Work out the finished part from the listing and answer in its coordinate system (mm). A direction names the side the tool comes from. Coordinates: 2 decimals unless noted, no trailing zeros. Order: outer loops, then holes, each group sorted by start corner. A loop starts at its lowest first (then second) coordinate and runs counter-clockwise, first axis right, second up. Notation, with made-up numbers: (32, 78) -> (72, 78) arc R24 cw to (72, 93) -> close; hole circle Ø4 at (89.25, 60). An arc over 180 degrees is marked (long way). Use one line per item in the form item = value.
from build123d import *

# Parameters (mm, degrees)
SKETCH1_W           = 37
SKETCH1_H           = 22.5
BOSS_EXTRUDE1_DEPTH = 20
BOSS_EXTRUDE2_DEPTH = 25
SKETCH3_R           = 2.5
BOSS_EXTRUDE3_DEPTH = 9.1
SKETCH4_R           = 2.5
BOSS_EXTRUDE4_DEPTH = 9.1
FILLET1_R           = 3
FILLET2_R           = 4
SKETCH5_W           = 2.75
SKETCH5_H           = 5
BOSS_EXTRUDE5_DEPTH = 5
SKETCH6_R           = 1.5
CUT_EXTRUDE1_DEPTH  = 2.75
SKETCH7_R           = 1.5
CUT_EXTRUDE2_DEPTH  = 30.1
SKETCH8_W           = 8.509980697
SKETCH8_H           = 2.764975678
SKETCH8_W_2         = 9.677414873
SKETCH8_H_2         = 2.427034206
CUT_EXTRUDE3_DEPTH  = 8.9
SKETCH9_W           = 9.677414873
SKETCH9_H           = 2.427034206
SKETCH9_W_2         = 8.509980697
SKETCH9_H_2         = 2.764975678
CUT_EXTRUDE4_DEPTH  = 8.9


with BuildPart() as part:
    # Sketch1 → Boss-Extrude1 (new body)
    with BuildSketch(Plane.XY):
        with Locations((-45.764100782, -13.75)):
            Rectangle(SKETCH1_W, SKETCH1_H)
    extrude(amount=-BOSS_EXTRUDE1_DEPTH)

    # Sketch2 → Boss-Extrude2 (add)
    with BuildSketch(Plane(origin=(-27.264100782, 0, 0), x_dir=(0, 0, -1), z_dir=(1, 0, 0))):
        with BuildLine():
            ThreePointArc((0.050125629, -14), (10, -24.462429423), (19.949874371, -14))
            ThreePointArc((19.949874371, -14), (10, -3), (0.050125629, -14))
        make_face()
    extrude(amount=BOSS_EXTRUDE2_DEPTH)

    # Sketch3 → Boss-Extrude3 (add)
    with BuildSketch(Plane.XY):
        with Locations((-54.264100782, -14)):
            Circle(SKETCH3_R)
    extrude(amount=BOSS_EXTRUDE3_DEPTH)

    # Sketch4 → Boss-Extrude4 (add)
    with BuildSketch(Plane(origin=(0, 0, -20), x_dir=(-1, 0, 0), z_dir=(0, 0, -1))):
        with Locations((54.264100782, -14)):
            Circle(SKETCH4_R)
    extrude(amount=BOSS_EXTRUDE4_DEPTH)

    # Fillet1
    fillet1_edges = [part.edges().sort_by_distance(p)[0] for p in [
        (-64.264100782, -2.5, -10),
        (-64.264100782, -25, -10),
    ]]
    fillet(fillet1_edges, radius=FILLET1_R)

    # Fillet2
    fillet2_edges = [part.edges().sort_by_distance(p)[0] for p in [
        (-2.264100782, -3, -10),
        (-2.264100782, -24.462429423, -10),
    ]]
    fillet(fillet2_edges, radius=FILLET2_R)

    # Sketch5 → Boss-Extrude5 (add)
    with BuildSketch(Plane.ZY.offset(64.264100782)):
        with Locations((-10, -13.75)):
            Rectangle(SKETCH5_W, SKETCH5_H)
    extrude(amount=BOSS_EXTRUDE5_DEPTH)

    # Sketch6 → Cut-Extrude1 (cut)
    with BuildSketch(Plane(origin=(0, 0, -11.375), x_dir=(-1, 0, 0), z_dir=(0, 0, -1))):
        with Locations((66.764100782, -13.75)):
            Circle(SKETCH6_R)
    extrude(amount=-CUT_EXTRUDE1_DEPTH, mode=Mode.SUBTRACT)

    # Sketch7 → Cut-Extrude2 (cut, through all)
    with BuildSketch(Plane(origin=(0, 0, -20), x_dir=(-1, 0, 0), z_dir=(0, 0, -1))):
        with Locations((31.264100782, -5)):
            Circle(SKETCH7_R)
        with Locations((31.264100782, -23)):
            Circle(SKETCH7_R)
    extrude(amount=-CUT_EXTRUDE2_DEPTH, mode=Mode.SUBTRACT)

    # Sketch8 → Cut-Extrude3 (cut)
    with BuildSketch(Plane(origin=(0, 0, -29.1), x_dir=(-1, 0, 0), z_dir=(0, 0, -1))):
        with Locations((54.477604306, -17.132487839)):
            Rectangle(SKETCH8_W, SKETCH8_H)
        with Locations((54.323994545, -11.036482897)):
            Rectangle(SKETCH8_W_2, SKETCH8_H_2)
    extrude(amount=-CUT_EXTRUDE3_DEPTH, mode=Mode.SUBTRACT)

    # Sketch9 → Cut-Extrude4 (cut)
    with BuildSketch(Plane.XY.offset(9.1)):
        with Locations((-54.323994545, -11.036482897)):
            Rectangle(SKETCH9_W, SKETCH9_H)
        with Locations((-54.477604306, -17.132487839)):
            Rectangle(SKETCH9_W_2, SKETCH9_H_2)
    extrude(amount=-CUT_EXTRUDE4_DEPTH, mode=Mode.SUBTRACT)


solid = part.part
(1) Which of the six approach directions +Z, -Z, +X, -X, +Y, -Y give full straight-line access (tool end or side, diameter ignored) to faces 1 (the cylindrical face through (-51.767, -13.89, -24.486)), 2 (the flat face through (-54, -12.25, 5)), 3 (the flat face through (-54, -15.75, -25)), 4 (the flat face through (-54, -15.75, 5))?
Data:
face_1 = -Z
face_2 = +Z, +X, -X, +Y
face_3 = -Z, +X, -X, -Y
face_4 = +Z, +X, -X, -Y
(2) Straight lines are drawn through the part: line 1 along Z through (x, y) = (-34, -19.75); line 2 along X through (y, z) = (-14, -15); line 3 along X through (y, z) = (-22.25, -10.5). For each, find the intervals that lie inside material, in ascending order.
Data:
line_1 = -20 to 0
line_2 = -64.26 to -2.26
line_3 = -64.25 to -32.56, -29.97 to -2.69
(3) Section A-A on z = -10 is taken. Write down the section's boundary in (x, y), plus the area to 3 significant figures.
Data:
outline = (-69.26, -16.25) -> (-64.26, -16.25) -> (-64.26, -22) arc R3 ccw to (-61.26, -25) -> (-27.26, -25) -> (-27.26, -24.46) -> (-6.26, -24.46) arc R4 ccw to (-2.26, -20.46) -> (-2.26, -7) arc R4 ccw to (-6.26, -3) -> (-27.26, -3) -> (-27.26, -2.5) -> (-61.26, -2.5) arc R3 ccw to (-64.26, -5.5) -> (-64.26, -11.25) -> (-69.26, -11.25) -> close; hole circle Ø3 at (-66.76, -13.75); hole circle Ø3 at (-31.26, -23); hole circle Ø3 at (-31.26, -5)
area = 1,360 mm²
(4) Section D-D on x = -58 is taken. Write down the section's boundary in (y, z).
Data:
outline = (-25, -20) -> (-2.5, -20) -> (-2.5, 0) -> (-25, 0) -> close
(5) Each of these flat-tipped pins is pushed along its axis until it touches: P1, Ø0.6, axis at x = -54.5, y = -16, coming from the -Z side; P2, Ø10, axis at x = -14, y = -7.5, coming from the +Z side; P3, Ø10, axis at y = -11, z = 3, coming from the +X side; P4, Ø7, axis at x = -41, y = -13, coming from the -Z side. Where does it stop, or does it pass through?
Data:
P1 = -29.1
P2 = -0.01
P3 = -2.89
P4 = -20
(6) Section C-C on z = -19 is taken. Count the separate pieces of the cut face and the enclosed holes in it, plus the area to 3 significant figures.
Data:
separate_pieces = 1
enclosed_holes = 2
area = 1,050 mm²
(7) Section B-B on x = -31.5 is taken. Write down the section's boundary in (y, z), plus the area to 3 significant figures.
Data:
outline = (-25, -20) -> (-24.48, -20) -> (-24.48, 0) -> (-25, 0) -> close; (-21.52, -20) -> (-6.48, -20) -> (-6.48, 0) -> (-21.52, 0) -> close; (-3.52, -20) -> (-2.5, -20) -> (-2.5, 0) -> (-3.52, 0) -> close
area = 331 mm²
